from build123d import *

# Parameters (mm, degrees)
SKETCH1_W           = 100
SKETCH1_H           = 500
BOSS_EXTRUDE1_DEPTH = 50
FILLET1_R           = 10
FILLET2_R           = 10
SKETCH2_R           = 40
BOSS_EXTRUDE2_DEPTH = 330


with BuildPart() as part:
    # Sketch1 → Boss-Extrude1 (new body)
    with BuildSketch(Plane(origin=(0, 0, 0), x_dir=(0, 0, -1), z_dir=(1, 0, 0))):
        with Locations((50, -250)):
            Rectangle(SKETCH1_W, SKETCH1_H)
    extrude(amount=BOSS_EXTRUDE1_DEPTH)

    # Fillet1
    fillet1_edges = [part.edges().sort_by_distance(p)[0] for p in [
        (50, 0, -50),
        (0, 0, -50),
        (0, -500, -50),
        (25, 0, 0),
        (25, 0, -100),
        (25, -500, -100),
        (25, -500, 0),
        (50, -500, -50),
    ]]
    fillet(fillet1_edges, radius=FILLET1_R)

    # Fillet2
    # the kernel refuses this fillet: 10 mm, written as the material it takes off along each edge
    with BuildSketch(Plane(origin=(40, -10, -10), x_dir=(0, 0, 1), z_dir=(1, 0, 0))) as fillet2_piece_1_section:
        Polygon((0, 0), (FILLET2_R, 0), (FILLET2_R, -FILLET2_R), (0, -FILLET2_R), align=None)
    fillet2_piece_1 = extrude(amount=FILLET2_R, mode=Mode.PRIVATE)
    fillet2_piece_1 = fillet2_piece_1 - Plane(origin=(40, -10, -10), x_dir=(0, -0.7071067811865475, -0.7071067811865476), z_dir=(1, 0, 0)) * Sphere(FILLET2_R, mode=Mode.PRIVATE)
    add(fillet2_piece_1, mode=Mode.SUBTRACT)
    with BuildSketch(Plane(origin=(40, -10, -90), x_dir=(0, 0, -1), z_dir=(1, 0, 0))) as fillet2_piece_2_section:
        Polygon((0, 0), (FILLET2_R, 0), (FILLET2_R, FILLET2_R), (0, FILLET2_R), align=None)
    fillet2_piece_2 = extrude(amount=FILLET2_R, mode=Mode.PRIVATE)
    fillet2_piece_2 = fillet2_piece_2 - Plane(origin=(40, -10, -90), x_dir=(0, -0.7071067811865477, 0.7071067811865475), z_dir=(1, 0, 0)) * Sphere(FILLET2_R, mode=Mode.PRIVATE)
    add(fillet2_piece_2, mode=Mode.SUBTRACT)
    with BuildSketch(Plane(origin=(40, -490, -10), x_dir=(0, 0, 1), z_dir=(1, 0, 0))) as fillet2_piece_3_section:
        Polygon((0, 0), (FILLET2_R, 0), (FILLET2_R, FILLET2_R), (0, FILLET2_R), align=None)
    fillet2_piece_3 = extrude(amount=FILLET2_R, mode=Mode.PRIVATE)
    fillet2_piece_3 = fillet2_piece_3 - Plane(origin=(40, -490, -10), x_dir=(0, 0.7071067811865477, -0.7071067811865475), z_dir=(1, 0, 0)) * Sphere(FILLET2_R, mode=Mode.PRIVATE)
    add(fillet2_piece_3, mode=Mode.SUBTRACT)
    with BuildSketch(Plane(origin=(40, -490, -90), x_dir=(0, 0, -1), z_dir=(1, 0, 0))) as fillet2_piece_4_section:
        Polygon((0, 0), (FILLET2_R, 0), (FILLET2_R, -FILLET2_R), (0, -FILLET2_R), align=None)
    fillet2_piece_4 = extrude(amount=FILLET2_R, mode=Mode.PRIVATE)
    fillet2_piece_4 = fillet2_piece_4 - Plane(origin=(40, -490, -90), x_dir=(0, 0.7071067811865475, 0.7071067811865476), z_dir=(1, 0, 0)) * Sphere(FILLET2_R, mode=Mode.PRIVATE)
    add(fillet2_piece_4, mode=Mode.SUBTRACT)
    with BuildSketch(Plane(origin=(50, -10, -100), x_dir=(0, 0, 1), z_dir=(0, -1, 0)), Plane(origin=(50, -490, 0), x_dir=(0, 0, -1), z_dir=(0, 1, 0))) as fillet2_piece_5:
        with BuildLine():
            CenterArc((FILLET2_R, FILLET2_R), FILLET2_R, 180, 90)
            Line((0, FILLET2_R), (0, 0))
            Line((0, 0), (FILLET2_R, 0))
        make_face()
    extrude(amount=480, mode=Mode.SUBTRACT)

    # Sketch2 → Boss-Extrude2 (add)
    with BuildSketch(Plane(origin=(50, 0, 0), x_dir=(0, 0, -1), z_dir=(1, 0, 0))):
        with Locations((50, -250)):
            Circle(SKETCH2_R)
    extrude(amount=BOSS_EXTRUDE2_DEPTH)


solid = part.part
Work out the finished part from the listing and answer in its coordinate system (mm). A direction names the side the tool comes from. Round coordinates to 2 decimals unless told otherwise and drop trailing zeros. Write each loop counter-clockwise with the first axis right and the second up, starting at its lowest first coordinate (ties: lowest second). Pieces come first, ordered by that corner, then holes. Notation, with made-up numbers: (28.5, -23.5) - (32.5, -23.5) arc R13 ccw to (32.5, -2.5) - close; hole circle Ø10 at (17, -27). An arc over 180 degrees is marked (long way). Answer in a Markdown table with one row per item. Add a question column.
1. Find the intervals of material crossed by line 1 along X through (y, z) = (-265, -91.5); line 2 along X through (y, z) = (-191, -18.5); line 3 along Y through (x, z) = (296, -33), in increasing order. Write a range as from..to.
2. For faces 1 (the cylindrical face through (20.28, -497.15, -96.99)), 2 (the cylindrical face through (212.69, -289.05, -41.33)), determine the directions among +Z, -Z, +X, -X, +Y, -Y from which every point of the face is accessible in a straight line to the end or side of a thin tool.
3. Given pin 1 (6 mm diameter, centred on x = 247.5, y = -248.5, fed in from -Z); pin 2 (2 mm diameter, centred on x = 222, y = -226, fed in from -Z); pin 3 (6 mm diameter, centred on x = 293.5, z = -18, fed in from -Y), each flat-ended and moving along its own axis, determine where each tip first touches the part or whether it passes through.
4. A cutting plane is placed at A-A, the plane z = -50. Determine the outline of the cut face in (x, y), and give its area (3 significant figures).
5. A cutting plane is placed at C-C, the plane x = 71. Determine the outline of the cut face in (y, z), and give its area (3 significant figures).
6. A cutting plane is placed at B-B, the plane y = -443.5. Determine the outline of the cut face in (x, z), and give its area (3 significant figures).
Worked out:
| question | item | result |
|---|---|---|
| 1 | line 1 | 0..49.89 |
| 1 | line 2 | 0..50 |
| 1 | line 3 | -286.21..-213.79 |
| 2 | face 1 | -Z, +X, -X, -Y |
| 2 | face 2 | +X |
| 3 | pin 1 | z = -90 |
| 3 | pin 2 | z = -82.73 |
| 3 | pin 3 | y = -277.55 |
| 4 | outline | (0, -490) arc R10 ccw to (10, -500) - (40, -500) arc R10 ccw to (50, -490) - (50, -290) - (380, -290) - (380, -210) - (50, -210) - (50, -10) arc R10 ccw to (40, 0) - (10, 0) arc R10 ccw to (0, -10) - close |
| 4 | area | 51,300 mm^2 |
| 5 | outline | circle Ø80 at (-250, -50) |
| 5 | area | 5,030 mm^2 |
| 6 | outline | (0, -100) - (40, -100) arc R10 ccw to (50, -90) - (50, -10) arc R10 ccw to (40, 0) - (0, 0) - close |
| 6 | area | 4,960 mm^2 |
